Input: dimensioned drawing with shaded views. Units: mm. Origin: part minimum x, y, z. A direction names the side the tool comes from. Give positions to 0.01 mm unless a question says otherwise; leave off trailing zeros. Loops run counter-clockwise (first coordinate to the right, second up) from the corner with the lowest first, then second, coordinate; pieces in that order, holes last.
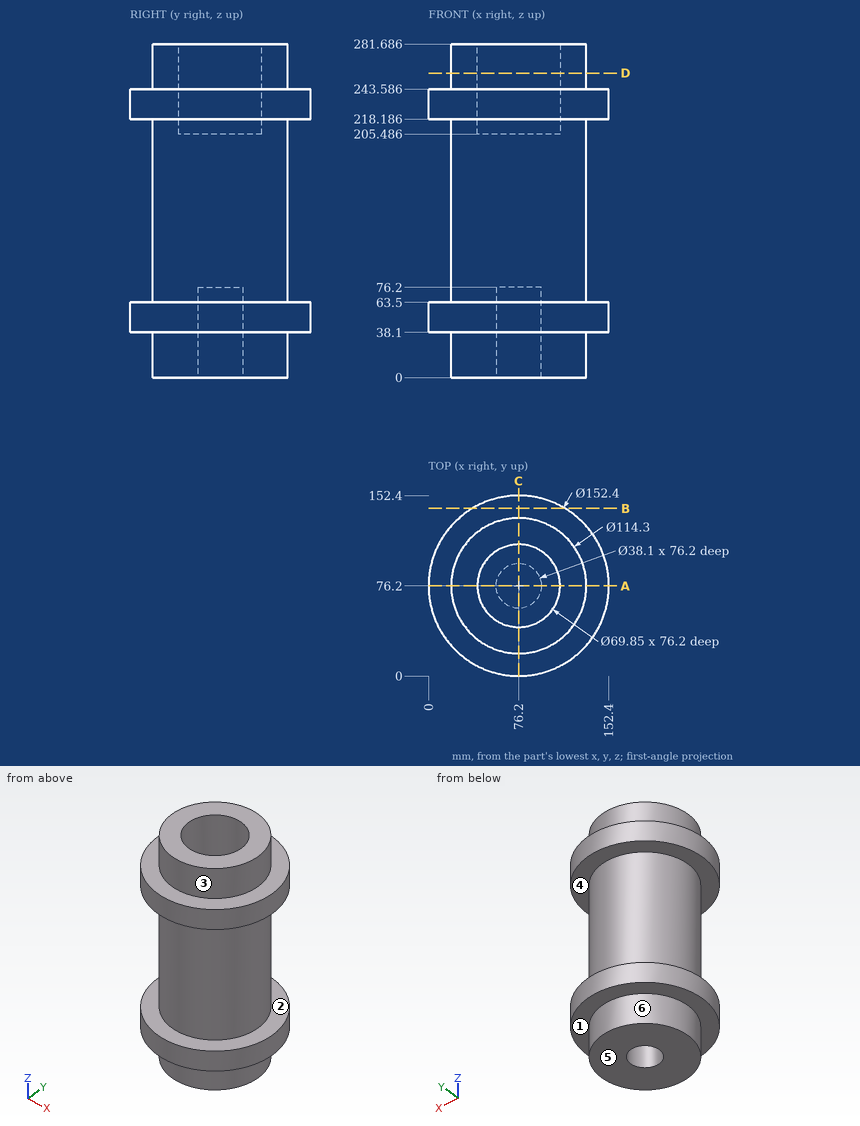
Item 1: Section query A-A on y = 76.2. Return loops of the section in (x, z) (3 decimals).
Values follow:
outline: (0, 38.1) - (19.05, 38.1) - (19.05, 0) - (57.15, 0) - (57.15, 76.2) - (95.25, 76.2) - (95.25, 0) - (133.35, 0) - (133.35, 38.1) - (152.4, 38.1) - (152.4, 63.5) - (133.35, 63.5) - (133.35, 218.186) - (152.4, 218.186) - (152.4, 243.586) - (133.35, 243.586) - (133.35, 281.686) - (111.125, 281.686) - (111.125, 205.486) - (41.275, 205.486) - (41.275, 281.686) - (19.05, 281.686) - (19.05, 243.586) - (0, 243.586) - (0, 218.186) - (19.05, 218.186) - (19.05, 63.5) - (0, 63.5) - close
Item 2: Draft query along Z for the marked faces 4, 5 and 6. Return one class per face: +Z half, -Z half, draft (parallel to the pull), parting line (faces both ways), or undercut.
Values follow:
face 4: undercut
face 5: -Z half
face 6: draft
Item 3: Section query D-D on z = 257. Return loops of the section in (x, y) (3 decimals).
Values follow:
outline: circle Ø114.3 at (76.2, 76.2); hole circle Ø69.85 at (76.2, 76.2)
Item 4: Ray query, probe 1 along Z at (x, y) = (11, 95); probe 2 along X at (y, z) = (76, 264); probe 3 along X at (y, z) = (76, 18). Return the intervals inside material, ascending.
Values follow:
probe 1: z = 38.1 to 63.5, 218.19 to 243.59
probe 2: x = 19.05 to 41.28, 111.12 to 133.35
probe 3: x = 19.05 to 57.15, 95.25 to 133.35
Item 5: Pin query (flat end, axial travel): pin 1 (12 mm diameter, centred on x = 123.5, y = 16.5, fed in from +Z); pin 2 (11.5 mm diameter, centred on x = 81.5, y = 72.5, fed in from -Z); pin 3 (8 mm diameter, centred on x = 96.5, z = 103, fed in from +Y). Return the tip coordinate at first contact, or that it passes through.
Values follow:
pin 1: stops at z = 243.59
pin 2: stops at z = 76.2
pin 3: stops at y = 130.98
Item 6: Section query B-B on y = 141.5. Return loops of the section in (x, z), plus the area to 3 significant figures.
Values follow:
outline: (36.93, 38.1) - (115.47, 38.1) - (115.47, 63.5) - (36.93, 63.5) - close; (36.93, 218.19) - (115.47, 218.19) - (115.47, 243.59) - (36.93, 243.59) - close
area: 3,990 mm2
Item 7: Set-up query: the marked faces 1, 2 and 3. Return all of +Z, -Z, +X, -X, +Y, -Y with unobstructed straight access to the full face (end or side cutting, diameter ignored); none if empty.
Values follow:
face 1: -Z
face 2: none
face 3: +Z
